```python
from build123d import *

# Parameters (mm, degrees)
F0_R      = 17
F1_DEPTH  = 62
F2_T      = -2
F3_W      = 2
F3_H      = 20
F4_DEPTH  = 25
F5_W      = 2
F5_H      = 20
F6_DEPTH  = 25
F7_W      = 2
F7_H      = 20
F8_DEPTH  = 25
F9_W      = 2
F9_H      = 20
F10_DEPTH = 25
F11_R     = 1.5
F12_DEPTH = 25
F13_R     = 1.5
F14_DEPTH = 25
F15_R     = 1.5
F16_DEPTH = 25
F17_R     = 1.5
F18_DEPTH = 25
F19_R     = 2
F20_DEPTH = 25


with BuildPart() as f1:
    # F0 (on Top) → F1 (new body)
    with BuildSketch(Plane.XY):
        Circle(F0_R)
    extrude(amount=F1_DEPTH)

    # F2
    f2_openings = [f1.faces().sort_by_distance(p)[0] for p in [
        (0, 0, 62),
    ]]
    offset(amount=F2_T, openings=f2_openings)

    # F3 (on Front) → F4 (cut)
    with BuildSketch(Plane.XZ):
        with Locations((0, 20)):
            Rectangle(F3_W, F3_H)
    extrude(amount=-F4_DEPTH, mode=Mode.SUBTRACT)

    # F5 (on Front) → F6 (cut)
    with BuildSketch(Plane.XZ):
        with Locations((0, 20)):
            Rectangle(F5_W, F5_H)
    extrude(amount=F6_DEPTH, mode=Mode.SUBTRACT)

    # F7 (on Right) → F8 (cut)
    with BuildSketch(Plane.YZ):
        with Locations((0, 20)):
            Rectangle(F7_W, F7_H)
    extrude(amount=-F8_DEPTH, mode=Mode.SUBTRACT)

    # F9 (on Right) → F10 (cut)
    with BuildSketch(Plane.YZ):
        with Locations((0, 20)):
            Rectangle(F9_W, F9_H)
    extrude(amount=F10_DEPTH, mode=Mode.SUBTRACT)

    # F11 (on Front) → F12 (cut)
    with BuildSketch(Plane.XZ):
        with Locations((7.5, 5)):
            Circle(F11_R)
        with Locations((-7.5, 5)):
            Circle(F11_R)
    extrude(amount=-F12_DEPTH, mode=Mode.SUBTRACT)

    # F13 (on Front) → F14 (cut)
    with BuildSketch(Plane.XZ):
        with Locations((7.5, 5)):
            Circle(F13_R)
        with Locations((-7.5, 5)):
            Circle(F13_R)
    extrude(amount=F14_DEPTH, mode=Mode.SUBTRACT)

    # F15 (on Right) → F16 (cut)
    with BuildSketch(Plane.YZ):
        with BuildLine():
            ThreePointArc((7.5, 3.5), (8.56066, 3.93934), (9, 5))
            ThreePointArc((9, 5), (6.43934, 6.06066), (7.5, 3.5))
        make_face()
        with Locations((-7.5, 5)):
            Circle(F15_R)
    extrude(amount=-F16_DEPTH, mode=Mode.SUBTRACT)

    # F17 (on Right) → F18 (cut)
    with BuildSketch(Plane.YZ):
        with Locations((-7.5, 5)):
            Circle(F17_R)
        with Locations((7.5, 5)):
            Circle(F17_R)
    extrude(amount=F18_DEPTH, mode=Mode.SUBTRACT)

    # F19 (on face) → F20 (cut)
    with BuildSketch(Plane(origin=(0, 0, 0), x_dir=(1, 0, 0), z_dir=(0, 0, -1))):
        Circle(F19_R)
    extrude(amount=-F20_DEPTH, mode=Mode.SUBTRACT)


solid = f1.part
```
Source: CAD feature listing. Evaluate the final solid. Frame: model axes, mm. A direction names the side the tool comes from. Give positions to 0.01 mm unless a question says otherwise; leave off trailing zeros. Loops run counter-clockwise (first coordinate to the right, second up) from the corner with the lowest first, then second, coordinate; pieces in that order, holes last. Notation, with made-up numbers: M 43,52 L 65,52 A27 ccw 65,91 Z; hole C 59,71 d6. An arc over 180 degrees is marked long. Put each result on its own line as item: value.
Q1. Section A-A (z = 16.5). Return the cut outline in (x, y), and give its area (3 significant figures).
Response values:
outline: M -16.97,-1 A17 ccw -1,-16.97 L -1,-14.97 A15 cw -14.97,-1 Z; M -16.97,1 L -14.97,1 A15 cw -1,14.97 L -1,16.97 A17 ccw Z; M 1,-16.97 A17 ccw 16.97,-1 L 14.97,-1 A15 cw 1,-14.97 Z; M 1,14.97 A15 cw 14.97,1 L 16.97,1 A17 ccw 1,16.97 Z
area: 185 mm²
Q2. Pin query (flat end, axial travel): P1, Ø3.5, axis at y = 7.5, z = 5, coming from the +X side; P2, Ø1, axis at y = 4, z = 29, coming from the -X side; P3, Ø2, axis at y = 3.5, z = 44.5, coming from the +X side; P4, Ø2.5, axis at y = 7.5, z = 5, coming from the -X side. Return the tip coordinate at first contact, or that it passes through.
Response values:
P1: stops at x = 16
P2: stops at x = -16.64
P3: stops at x = 16.82
P4: passes through
Q3. Section B-B (x = 0). Return the cut outline in (y, z), and give its area (3 significant figures).
Response values:
outline: M -17,0 L -2,0 L -2,2 L -15,2 L -15,10 L -17,10 Z; M -17,30 L -15,30 L -15,62 L -17,62 Z; M 2,0 L 17,0 L 17,10 L 15,10 L 15,2 L 2,2 Z; M 15,30 L 17,30 L 17,62 L 15,62 Z
area: 220 mm²
Q4. Mould query, pull axis X, two halves, no side actions, for faces 4 (the flat face through (1, -16, 20)), 5 (the flat face through (16, 0, 30)), 6 (the cylindrical face through (16.215, 5.106, 30.566)), 7 (the flat face through (1, 16, 20)). Classes: released by +X, released by -X, zero draft, split by the parting line, or undercut.
Response values:
face 4: undercut
face 5: zero draft
face 6: split by the parting line
face 7: undercut
Q5. Section D-D (x = 7.5). Return the cut outline in (y, z), and give its area (3 significant figures).
Response values:
outline: M -15.26,0 L 15.26,0 L 15.26,3.5 L 12.99,3.5 L 12.99,2 L -12.99,2 L -12.99,3.5 L -15.26,3.5 Z; M -15.26,6.5 L -12.99,6.5 L -12.99,62 L -15.26,62 Z; M 12.99,6.5 L 15.26,6.5 L 15.26,62 L 12.99,62 Z
area: 319 mm²
Q6. Line query: probe 1 along Y at (x, z) = (1, 9.5); probe 2 along Z at (x, y) = (-7.5, -14.45). Output: solid intervals per line, ascending. Write a range as [from, to].
Response values:
probe 1: y = [-16.97, -14.97], [14.97, 16.97]
probe 2: z = [0, 3.5], [6.5, 62]
Q7. Reachability of faces 1 (the flat face through (0, 16, 10)), 2 (the flat face through (16, -1, 20)), 3 (the flat face through (3, 0, 2)) from +Z, -Z, +X, -X, +Y, -Y: full face, straight path, thin tool, end or side. Return the list, or none.
Response values:
face 1: +Y, -Y
face 2: +X, -X
face 3: +Z
